```python
from build123d import *

# Parameters (mm, degrees)
SKETCH1_R             = 14
SKETCH1_R_2           = 5.1
BOSS_EXTRUDE1_DEPTH   = 15
M3_TAPPED_HOLE1_D     = 2.5
M3_TAPPED_HOLE1_DEPTH = 6.5
M3_TAPPED_HOLE1_TIP   = 0.751075774
M3_TAPPED_HOLE2_D     = 2.5
M3_TAPPED_HOLE2_DEPTH = 6.5
M3_TAPPED_HOLE2_TIP   = 0.751075774
SKETCH19_R            = 4
CUT_EXTRUDE3_DEPTH    = 7
CIRPATTERN2_COUNT     = 3


with BuildPart() as part:
    # Sketch1 → Boss-Extrude1 (new body)
    with BuildSketch(Plane.XY):
        Circle(SKETCH1_R)
        Circle(SKETCH1_R_2, mode=Mode.SUBTRACT)
    extrude(amount=BOSS_EXTRUDE1_DEPTH)

    # M3 Tapped Hole1
    with Locations(Plane.XY.offset(15)):
        with Locations((0, -8), (-8, 0), (0, 8), (8, 0)):
            Hole(M3_TAPPED_HOLE1_D / 2, depth=M3_TAPPED_HOLE1_DEPTH)
            with Locations((0, 0, -(M3_TAPPED_HOLE1_DEPTH + M3_TAPPED_HOLE1_TIP / 2))):  # 118° drill point
                Cone(0, M3_TAPPED_HOLE1_D / 2, M3_TAPPED_HOLE1_TIP, mode=Mode.SUBTRACT)

    # M3 Tapped Hole2
    with Locations(Plane(origin=(0, 0, 0), x_dir=(-1, 0, 0), z_dir=(0, 0, -1))):
        with Locations((0, -10.5), (-9.09326674, 5.25), (9.09326674, 5.25)):
            Hole(M3_TAPPED_HOLE2_D / 2, depth=M3_TAPPED_HOLE2_DEPTH)
            with Locations((0, 0, -(M3_TAPPED_HOLE2_DEPTH + M3_TAPPED_HOLE2_TIP / 2))):  # 118° drill point
                Cone(0, M3_TAPPED_HOLE2_D / 2, M3_TAPPED_HOLE2_TIP, mode=Mode.SUBTRACT)

    # Sketch19 → Cut-Extrude3 (cut)
    with BuildSketch(Plane(origin=(14, 0, 0), x_dir=(0, 0, -1), z_dir=(1, 0, 0))):
        with Locations((-7.5, 5.25)):
            Circle(SKETCH19_R)
    cut_extrude3 = extrude(amount=-CUT_EXTRUDE3_DEPTH, mode=Mode.SUBTRACT)

    # CirPattern2: Cut-Extrude3 ×3 about axis
    cirpattern2_axis = Axis((0, 0, 0), (0, 0, 1))
    for i in range(1, CIRPATTERN2_COUNT):
        add(cut_extrude3.rotate(cirpattern2_axis, i * 360 / CIRPATTERN2_COUNT), mode=Mode.SUBTRACT)


solid = part.part
```
Design review of the part built by this model. Coordinates are the model's own, in mm. A direction names the side the tool comes from. Round coordinates to 2 decimals unless told otherwise and drop trailing zeros. Order: outer loops, then holes, each group sorted by start corner. A loop starts at its lowest first (then second) coordinate and runs counter-clockwise, first axis right, second up. Notation, with made-up numbers: (34, -12) - (40, -12) arc R33 cw to (40, 23) - close; hole circle Ø3 at (13, -38.5). An arc over 180 degrees is marked (long way). Return JSON: item names as keys, results as strings.
Q1. Consider section C-C on z = 9.25. Write out the cut boundary in (x, y), plus the area to 3 significant figures.
Computed values:
{"outline": "(-13.09, 4.97) arc R14 ccw to (-5.52, -12.87) - (-2.07, -6.89) - (-1.12, -7.44) arc R1.25 cw (long way) to (1.04, -8.69) - (4.16, -10.49) - (2.24, -13.82) arc R14 ccw to (13.9, 1.65) - (7, 1.65) - (7, 8.85) - (10.85, 8.85) arc R14 ccw to (-8.38, 11.21) - (-4.93, 5.24) - (-11.16, 1.64) - close; hole circle Ø2.5 at (-8, 0); hole circle Ø10.2 at (0, 0); hole circle Ø2.5 at (0, 8); hole circle Ø2.5 at (8, 0)", "area": "392 mm2"}
Q2. The part is to be moulded in two halves that separate along X. For faces 5 (the cylindrical face through (-7.901, 5.625, 1.876)), 6 (the cylindrical face through (12.932, -5.362, 7.395)), 7 (the flat face through (7, 5, 8)), say which applies: pulls with the +X half, pulls with the -X half, needs draft (parallel to the pull), parting line crosses it, or undercut.
Computed values:
{"face 5": "undercut", "face 6": "parting line crosses it", "face 7": "pulls with the +X half"}
Q3. Machinability: for faces 1 (the flat face through (1.1, -8.72, 7.56)), 2 (the cylindrical face through (-6.75, 0.05, 11.7)), 3 (the cylindrical face through (9.67, 4.14, 1.88)), 4 (the cylindrical face through (9.749, 1.345, 8.367)), which of the approach directions +Z, -Z, +X, -X, +Y, -Y give a long, thin tool a straight path to every point of the face, cutting with its end or side? Answer none if there is none.
Computed values:
{"face 1": "none", "face 2": "+Z", "face 3": "-Z", "face 4": "+X"}
Q4. For pin 1 Ø5 at (y, z) = (-3, 2) entering from +X; pin 2 Ø6 at (y, z) = (-9.5, 3) entering from +X; pin 3 Ø9 at (x, y) = (0, 0) entering from +Z; pin 4 Ø5 at (x, z) = (10, 2) entering from -Y, all flat-tipped, find the tip position at first contact; note any pin that passes through.
Computed values:
{"pin 1": "stops at x = 13.99", "pin 2": "stops at x = 12.4", "pin 3": "passes through", "pin 4": "stops at y = -11.82"}
Q5. Consider section D-D on z = 1. Write out the cut boundary in (x, y), plus the area to 3 significant figures.
Computed values:
{"outline": "circle Ø28 at (0, 0); hole circle Ø2.5 at (-9.09, 5.25); hole circle Ø10.2 at (0, 0); hole circle Ø2.5 at (0, -10.5); hole circle Ø2.5 at (9.09, 5.25)", "area": "519 mm2"}
Q6. Consider section A-A on z = 12.25. Write out the cut boundary in (x, y), plus the area to 3 significant figures.
Computed values:
{"outline": "circle Ø28 at (0, 0); hole circle Ø2.5 at (-8, 0); hole circle Ø10.2 at (0, 0); hole circle Ø2.5 at (0, -8); hole circle Ø2.5 at (0, 8); hole circle Ø2.5 at (8, 0)", "area": "514 mm2"}
Q7. Consider section B-B on y = -4.25. Write out the cut boundary in (x, z).
Computed values:
{"outline": "(-13.34, 0) - (-2.82, 0) - (-2.82, 15) - (-13.34, 15) - close; (2.82, 0) - (13.34, 0) - (13.34, 15) - (2.82, 15) - close"}
Q8. Wall thickness on L1, parallel to Y at x = 0, z = 2.7; L2, parallel to X at y = 4.25, z = 5.25; L3, parallel to X at y = 4.5, z = 1.5: over which ranges is each line inside the solid? List them lowest first. Write a range as [from, to].
Computed values:
{"L1": "y = [-14, -11.75], [-9.25, -5.1], [5.1, 14]", "L2": "x = [-13.34, -12.33], [-6.64, -2.82], [2.82, 7]", "L3": "x = [-13.26, -10.09], [-8.09, -2.4], [2.4, 8.09], [10.09, 13.26]"}
